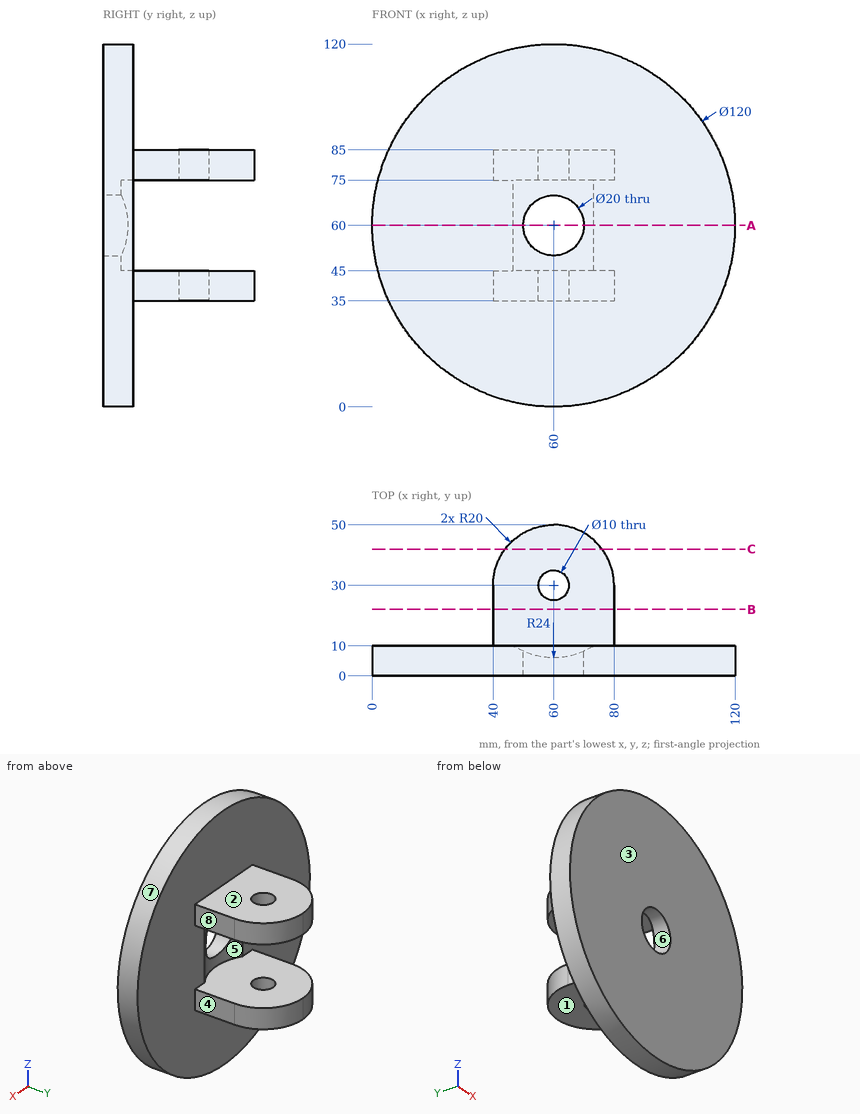
Could you check a few things on this drawing? It's one solid part, dimensions in mm from its lowest x, y, z. A direction names the side the tool comes from. Coordinates: 2 decimals unless noted, no trailing zeros. Write each loop counter-clockwise with the first axis right and the second up, starting at its lowest first coordinate (ties: lowest second). Pieces come first, ordered by that corner, then holes. Notation, with made-up numbers: (-36.5, 58) - (-14.5, 58) arc R25 cw to (-14.5, 95) - close; hole circle Ø4 at (-28, -6). An arc over 180 degrees is marked (long way). Return JSON: item names as keys, results as strings. Group by question number.
Item 1: If we section it at A-A (z = 60): Write out the boundary of the cut face in (x, y).
Item 2: If we section it at B-B (y = 22): Write out the boundary of the cut face in (x, z), then the cut area to 3 significant figures.
Item 3: Please list where these lines run through material, in increasing order: probe 1 along Z at (x, y) = (53.5, 36.5); probe 2 along X at (y, z) = (2.25, 60); probe 3 along Y at (x, z) = (60, 81).
Item 4: If we section it at C-C (y = 42): Write out the boundary of the cut face in (x, z).
Item 5: I'm going to push flat-ended pins straight in: pin 1 Ø1.5 at (x, z) = (44, 19) entering from +Y; pin 2 Ø12 at (x, y) = (63, 21.5) entering from -Z; pin 3 Ø1 at (x, y) = (54, 12.5) entering from +Z. Where does each tip first touch, or does it pass through?
Item 6: Which directions (+Z, -Z, +X, -X, +Y, -Y) give clear straight access to the entire face, cutting with the end or side of a thin tool? Please do the marked faces 1, 2, 3, 4 and 5.
Item 7: We'd pull the mould along Z, two halves only. Please class the marked faces 6, 7 and 8: pulls with the +Z half, pulls with the -Z half, needs draft (parallel to the pull), parting line crosses it, or undercut.
Return value:
{
 "1": {"outline": "(0, 0) - (50, 0) - (50, 8.18) arc R24 cw to (46.73, 10) - (0, 10) - close; (70, 0) - (120, 0) - (120, 10) - (73.27, 10) arc R24 cw to (70, 8.18) - close"},
 "2": {"outline": "(40, 35) - (80, 35) - (80, 45) - (40, 45) - close; (40, 75) - (80, 75) - (80, 85) - (40, 85) - close", "area": "800 mm^2"},
 "3": {"probe 1": "z = 35 to 45, 75 to 85", "probe 2": "x = 0 to 50, 70 to 120", "probe 3": "y = 0 to 25, 35 to 50"},
 "4": {"outline": "(44, 35) - (76, 35) - (76, 45) - (44, 45) - close; (44, 75) - (76, 75) - (76, 85) - (44, 85) - close"},
 "5": {"pin 1": "stops at y = 10", "pin 2": "stops at z = 35", "pin 3": "stops at z = 85"},
 "6": {"face 1": "-Z, +X, -X, +Y", "face 2": "+Z, +X, -X, +Y", "face 3": "+Z, -Z, +X, -X, -Y", "face 4": "+Z, -Z, +X, +Y", "face 5": "+Y"},
 "7": {"face 6": "undercut", "face 7": "parting line crosses it", "face 8": "needs draft"}
}
